Check sheet for the modelled part. Datum: model origin and axes. Units: mm. Face numbers are marked on the shaded views. A direction names the side the tool comes from. Round coordinates to 2 decimals unless told otherwise and drop trailing zeros. Order: outer loops, then holes, each group sorted by start corner. A loop starts at its lowest first (then second) coordinate and runs counter-clockwise, first axis right, second up. Notation, with made-up numbers: (-36, -37) -> (-10, -37) arc R15 ccw to (-10, -33) -> close; hole circle Ø8 at (34.25, -9.75). An arc over 180 degrees is marked (long way). Answer in a Markdown table with one row per item.
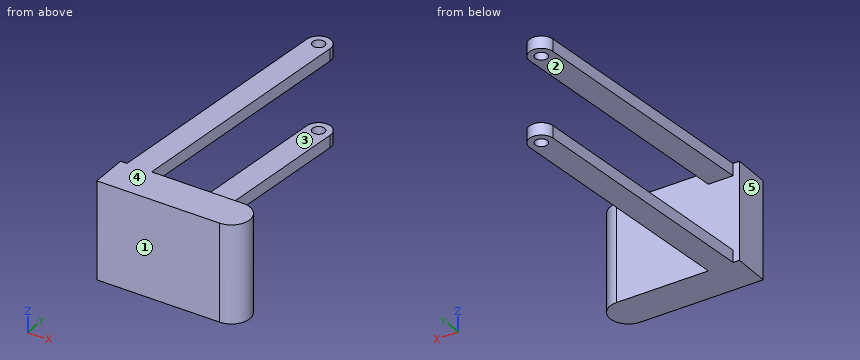
from build123d import *

# Parameters (mm, degrees)
SKETCH_1_R          = 0.5
EXTRUDE_1_DEPTH     = 8
SKETCH_2_W          = 6
SKETCH_2_H          = 21
CUT_EXTRUDE_1_DEPTH = 7


with BuildPart() as part:
    # 草圖1 → 填料-伸長1 (new body)
    with BuildSketch(Plane.XY):
        with BuildLine():
            Line((0.519160932, 3), (2.196426588, 23.083226007))
            ThreePointArc((2.196426588, 23.083226007), (3.276183293, 23.996530698), (4.189487983, 22.916773993))
            Line((4.189487983, 22.916773993), (2.526123692, 3))
            Line((2.526123692, 3), (10, 3))
            ThreePointArc((10, 3), (11.5, 1.5), (10, 0))
            Line((10, 0), (0, 0))
            Line((0, 0), (0, 3))
            Line((0, 3), (0.519160932, 3))
        make_face()
        with Locations((3.192957285, 23)):
            Circle(SKETCH_1_R, mode=Mode.SUBTRACT)
    extrude(amount=EXTRUDE_1_DEPTH)

    # 草圖2 → 除料-伸長1 (cut)
    with BuildSketch(Plane.ZY):
        with Locations((4, 13.5)):
            Rectangle(SKETCH_2_W, SKETCH_2_H)
    extrude(amount=-CUT_EXTRUDE_1_DEPTH, mode=Mode.SUBTRACT)


solid = part.part
Item 1: Cross-section at C-C (y = 3.25). Record the boundary of the cut face in (x, z).
Result sheet:
| item | result |
|---|---|
| outline | (0.54, 0) -> (2.55, 0) -> (2.55, 1) -> (0.54, 1) -> close; (0.54, 7) -> (2.55, 7) -> (2.55, 8) -> (0.54, 8) -> close |
Item 2: Scan lines: line 1 (Z direction, x = 2, y = 14); line 2 (Y direction, x = 4.25, z = 5.5); line 3 (X direction, y = 23, z = 0.3). Record each from-to range of solid material in increasing order. Write a range as [from, to].
Result sheet:
| item | result |
|---|---|
| line 1 | z = [0, 1], [7, 8] |
| line 2 | y = [0, 3] |
| line 3 | x = [2.19, 2.69], [3.69, 4.19] |
Item 3: Set-up check for the marked faces 1 and 2: record each of +Z, -Z, +X, -X, +Y, -Y from which the full face is reachable in a straight line by a thin tool's end or side.
Result sheet:
| item | result |
|---|---|
| face 1 | +Z, -Z, +X, -X, -Y |
| face 2 | +X, -X, +Y |
Item 4: Cross-section at B-B (x = 3). Record the boundary of the cut face in (y, z).
Result sheet:
| item | result |
|---|---|
| outline | (0, 0) -> (3, 0) -> (3, 8) -> (0, 8) -> close; (8.67, 0) -> (22.54, 0) -> (22.54, 1) -> (8.67, 1) -> close; (8.67, 7) -> (22.54, 7) -> (22.54, 8) -> (8.67, 8) -> close; (23.46, 0) -> (23.98, 0) -> (23.98, 1) -> (23.46, 1) -> close; (23.46, 7) -> (23.98, 7) -> (23.98, 8) -> (23.46, 8) -> close |
Item 5: Cross-section at D-D (x = 1.75). Record the boundary of the cut face in (y, z), and give its area (3 significant figures).
Result sheet:
| item | result |
|---|---|
| outline | (0, 0) -> (17.74, 0) -> (17.74, 1) -> (3, 1) -> (3, 7) -> (17.74, 7) -> (17.74, 8) -> (0, 8) -> close |
| area | 53.5 mm^2 |
Item 6: Cross-section at A-A (z = 0.75). Record the boundary of the cut face in (x, y).
Result sheet:
| item | result |
|---|---|
| outline | (0, 0) -> (10, 0) arc R1.5 ccw to (10, 3) -> (2.53, 3) -> (4.19, 22.92) arc R1 ccw to (2.2, 23.08) -> (0.52, 3) -> (0, 3) -> close; hole circle Ø1 at (3.19, 23) |
Item 7: Mould release check, pull along Z, two halves, no side actions. Record for the marked faces 3, 4 and 5: pulls with the +Z half, pulls with the -Z half, needs draft (parallel to the pull), parting line crosses it, or undercut.
Result sheet:
| item | result |
|---|---|
| face 3 | undercut |
| face 4 | pulls with the +Z half |
| face 5 | needs draft |
Item 8: Depth check by flat-ended pin: P1, Ø2, axis at x = 8.5, z = 2, coming from the +Y side. Enter the tip coordinate at first touch or a pass-through.
Result sheet:
| item | result |
|---|---|
| P1 | stops at y = 3 |
